The listing builds one solid part. Answer for the finished solid, in the listing's coordinates (mm). Face numbers are marked on the shaded views. A direction names the side the tool comes from. Coordinates: 2 decimals unless noted, no trailing zeros. Loops run counter-clockwise (first coordinate to the right, second up) from the corner with the lowest first, then second, coordinate; pieces in that order, holes last. Notation, with made-up numbers: (81.5, -3) - (114.5, -3) arc R30 cw to (114.5, 34) - close; hole circle Ø9 at (-27.5, 78). An arc over 180 degrees is marked (long way). Write each question's results on one line, items separated by ' | '. Start each with the question number.
(1) Find section B-B on z = 27. Determine the outline of the cut face in (x, y), then the cut area to 3 significant figures.
(2) Consider line 1 (Z direction, x = -3.25, y = 2.5); line 2 (Y direction, x = 4, z = 44.5); line 3 (Z direction, x = -7, y = 12.5). Determine where each line is inside the solid, lowest interval first. Write a range as from..to.
(3) For the marked faces 4, 5 and 6, determine the directions among +Z, -Z, +X, -X, +Y, -Y from which every point of the face is accessible in a straight line to the end or side of a thin tool.
(4) Find section A-A on x = 0. Determine the outline of the cut face in (y, z).
(5) Determine the mould class of the marked faces 1, 2 and 3 for opening direction Z: released by +Z, released by -Z, zero draft, split by the parting line, or undercut.
(6) Given pin 1 Ø11.5 at (x, y) = (-5, 10.5) entering from +Z; pin 2 Ø1 at (y, z) = (6, 38.5) entering from +X; pin 3 Ø2 at (x, z) = (2.5, 22) entering from +Y, each flat-ended and moving along its own axis, determine where each tip first touches the part or whether it passes through.
(7) Find section C-C on x = -8. Determine the outline of the cut face in (y, z).
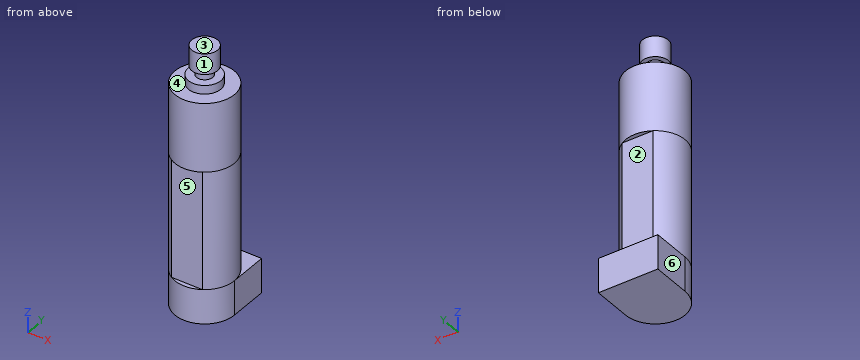
from build123d import *

# Parameters (mm, degrees)
BOSS_EXTRUDE1_DEPTH = 12.7
BOSS_EXTRUDE2_DEPTH = 43.434
SKETCH3_R           = 10.9855
BOSS_EXTRUDE3_DEPTH = 25.4
SKETCH4_R           = 6.0071
BOSS_EXTRUDE4_DEPTH = 3.175
SKETCH5_R           = 2.9972
BOSS_EXTRUDE5_DEPTH = 3.175
SKETCH6_R           = 4.7625
BOSS_EXTRUDE6_DEPTH = 7.62


with BuildPart() as part:
    # Sketch1 → Boss-Extrude1 (new body)
    with BuildSketch(Plane.XY):
        with BuildLine():
            Line((-10.9855, 0), (-10.9855, 14.4145))
            Line((-10.9855, 14.4145), (10.9855, 14.4145))
            Line((10.9855, 14.4145), (10.9855, 0))
            ThreePointArc((10.9855, 0), (0, -10.9855), (-10.9855, 0))
        make_face()
    extrude(amount=BOSS_EXTRUDE1_DEPTH)

    # Sketch2 → Boss-Extrude2 (add)
    with BuildSketch(Plane.XY.offset(12.7)):
        with BuildLine():
            Line((-5.68848, 9.398), (5.68848, 9.398))
            ThreePointArc((5.68848, 9.398), (10.9855, 0), (5.68848, -9.398))
            Line((5.68848, -9.398), (-5.68848, -9.398))
            ThreePointArc((-5.68848, -9.398), (-10.9855, 0), (-5.68848, 9.398))
        make_face()
    extrude(amount=BOSS_EXTRUDE2_DEPTH)

    # Sketch3 → Boss-Extrude3 (add)
    with BuildSketch(Plane.XY.offset(56.134)):
        Circle(SKETCH3_R)
    extrude(amount=BOSS_EXTRUDE3_DEPTH)

    # Sketch4 → Boss-Extrude4 (add)
    with BuildSketch(Plane.XY.offset(81.534)):
        Circle(SKETCH4_R)
    extrude(amount=BOSS_EXTRUDE4_DEPTH)

    # Sketch5 → Boss-Extrude5 (add)
    with BuildSketch(Plane.XY.offset(84.709)):
        Circle(SKETCH5_R)
    extrude(amount=BOSS_EXTRUDE5_DEPTH)

    # Sketch6 → Boss-Extrude6 (add)
    with BuildSketch(Plane.XY.offset(87.884)):
        Circle(SKETCH6_R)
    extrude(amount=BOSS_EXTRUDE6_DEPTH)


solid = part.part
Values:
1) outline: (-5.69, -9.4) - (5.69, -9.4) arc R10.99 ccw to (5.69, 9.4) - (-5.69, 9.4) arc R10.99 ccw to start | area: 355 mm²
2) line 1: z = 0..84.71, 87.88..95.5 | line 2: y = -9.4..9.4 | line 3: z = 0..12.7
3) face 4: +Z | face 5: +X, -X, -Y | face 6: +Z, -Z, -X, +Y, -Y
4) outline: (-10.99, 0) - (14.41, 0) - (14.41, 12.7) - (9.4, 12.7) - (9.4, 56.13) - (10.99, 56.13) - (10.99, 81.53) - (6.01, 81.53) - (6.01, 84.71) - (3, 84.71) - (3, 87.88) - (4.76, 87.88) - (4.76, 95.5) - (-4.76, 95.5) - (-4.76, 87.88) - (-3, 87.88) - (-3, 84.71) - (-6.01, 84.71) - (-6.01, 81.53) - (-10.99, 81.53) - (-10.99, 56.13) - (-9.4, 56.13) - (-9.4, 12.7) - (-10.99, 12.7) - close
5) face 1: zero draft | face 2: undercut | face 3: released by +Z
6) pin 1: stops at z = 84.71 | pin 2: stops at x = 9.51 | pin 3: stops at y = 9.4
7) outline: (-7.53, 0) - (14.41, 0) - (14.41, 12.7) - (7.53, 12.7) - (7.53, 81.53) - (-7.53, 81.53) - close
